Input: part model. Units: mm. Frame: model coordinates. A direction names the side the tool comes from. Give positions to 0.01 mm unless a question says otherwise; leave off trailing zeros. Order: outer loops, then holes, each group sorted by start corner. A loop starts at its lowest first (then second) coordinate and runs counter-clockwise, first axis right, second up. Notation, with made-up numbers: M 6.25,84.25 L 31.25,84.25 A27 ccw 31.25,108.25 Z; hole C 6,59 d8. An arc over 180 degrees is marked long. Use a Markdown table: item, result.
from build123d import *

# Parameters (mm, degrees)
SKETCH_1_W                 = 52.7
SKETCH_1_H                 = 13.9
EXTRUDE_1_DEPTH            = 11
SKETCH_2_W                 = 46.7
SKETCH_2_H                 = 10.9
CUT_EXTRUDE_1_DEPTH        = 9.5
SKETCH_3_W                 = 45.5
SKETCH_3_H                 = 1.5
EXTRUDE_2_DEPTH            = 8.4
SKETCH_4_W                 = 1
SKETCH_4_H                 = 7.5
CUT_EXTRUDE_2_DEPTH        = 51.794807806
CUT_EXTRUDE_3_DEPTH        = 3
PATTERN_LINEAR_1_COUNT     = 4
PATTERN_LINEAR_1_PITCH     = 5
CUT_EXTRUDE_4_DEPTH        = 3
PATTERN_LINEAR_2_COUNT     = 4
PATTERN_LINEAR_2_PITCH     = 5
SKETCH_7_W                 = 3.6
SKETCH_7_H                 = 5.5
CUT_EXTRUDE_5_DEPTH        = 32.757400712
SKETCH_8_W                 = 50.7
SKETCH_8_H                 = 11.9
CUT_EXTRUDE_6_DEPTH        = 0.5
SKETCH_9_R                 = 2.1
CUT_EXTRUDE_7_DEPTH        = 5
PATTERN_LINEAR_3_COUNT     = 5
PATTERN_LINEAR_3_PITCH     = 5.08
PATTERN_LINEAR_3_COL_COUNT = 5
PATTERN_LINEAR_3_COL_PITCH = 5.08
SKETCH_10_W                = 47.5
SKETCH_10_H                = 2
CUT_EXTRUDE_8_DEPTH        = 3
CUT_EXTRUDE_9_DEPTH        = 3


with BuildPart() as part:
    # Эскиз1 → Бобышка-Вытянуть1 (new body)
    with BuildSketch(Plane(origin=(0, 0, 0), x_dir=(1, 0, 0), z_dir=(0, 1, 0))):
        Rectangle(SKETCH_1_W, SKETCH_1_H)
    extrude(amount=EXTRUDE_1_DEPTH)

    # Эскиз2 → Вырез-Вытянуть1 (cut)
    with BuildSketch(Plane.XZ):
        Rectangle(SKETCH_2_W, SKETCH_2_H)
    extrude(amount=-CUT_EXTRUDE_1_DEPTH, mode=Mode.SUBTRACT)

    # Эскиз3 → Бобышка-Вытянуть2 (add)
    with BuildSketch(Plane.XZ):
        with Locations((0, 6.2)):
            Rectangle(SKETCH_3_W, SKETCH_3_H)
    extrude(amount=EXTRUDE_2_DEPTH)

    # Эскиз4 → Вырез-Вытянуть2 (cut, through all)
    with BuildSketch(Plane(origin=(22.75, 0, 0), x_dir=(0, 0, -1), z_dir=(1, 0, 0))):
        with Locations((-6.75, -5.15)):
            Rectangle(SKETCH_4_W, SKETCH_4_H)
    extrude(amount=-CUT_EXTRUDE_2_DEPTH, mode=Mode.SUBTRACT)

    # Эскиз5 → Вырез-Вытянуть3 (cut)
    with BuildSketch(Plane.XY.offset(6.25)):
        Polygon((-2.675, -1.4), (-2.675, -8), (-3.175, -8.5), (-3.675, -8.5), (-3.675, -9.5), (-1.375, -9.5), (-1.375, -8.5), (-1.875, -8.5), (-2.375, -8), (-2.375, -1.4), align=None)
    cut_extrude_3 = extrude(amount=-CUT_EXTRUDE_3_DEPTH, mode=Mode.SUBTRACT)

    # Линейный массив1: Вырез-Вытянуть3 ×4
    with Locations(*[(-i * PATTERN_LINEAR_1_PITCH, 0, 0) for i in range(1, PATTERN_LINEAR_1_COUNT)]):
        add(cut_extrude_3, mode=Mode.SUBTRACT)

    # Эскиз6 → Вырез-Вытянуть4 (cut)
    with BuildSketch(Plane.XY.offset(6.25)):
        Polygon((2.375, -1.4), (2.675, -1.4), (2.675, -8), (3.175, -8.5), (3.675, -8.5), (3.675, -9), (1.375, -9), (1.375, -8.5), (1.875, -8.5), (2.375, -8), align=None)
    cut_extrude_4 = extrude(amount=-CUT_EXTRUDE_4_DEPTH, mode=Mode.SUBTRACT)

    # Линейный массив2: Вырез-Вытянуть4 ×4
    with Locations(*[(i * PATTERN_LINEAR_2_PITCH, 0, 0) for i in range(1, PATTERN_LINEAR_2_COUNT)]):
        add(cut_extrude_4, mode=Mode.SUBTRACT)

    # Эскиз7 → Вырез-Вытянуть5 (cut, through all)
    with BuildSketch(Plane.XY.offset(6.95)):
        with Locations((-24.55, 1.75)):
            Rectangle(SKETCH_7_W, SKETCH_7_H)
        with Locations((24.55, 1.75)):
            Rectangle(SKETCH_7_W, SKETCH_7_H)
    extrude(amount=-CUT_EXTRUDE_5_DEPTH, mode=Mode.SUBTRACT)

    # Эскиз8 → Вырез-Вытянуть6 (cut)
    with BuildSketch(Plane(origin=(0, 11, 0), x_dir=(1, 0, 0), z_dir=(0, 1, 0))):
        Rectangle(SKETCH_8_W, SKETCH_8_H)
    extrude(amount=-CUT_EXTRUDE_6_DEPTH, mode=Mode.SUBTRACT)

    # Эскиз9 → Вырез-Вытянуть7 (cut)
    with BuildSketch(Plane(origin=(0, 10.5, 0), x_dir=(1, 0, 0), z_dir=(0, 1, 0))):
        with Locations(Location((0, 0, 0), (0, 0, 270))):
            Circle(SKETCH_9_R)
    cut_extrude_7 = extrude(amount=-CUT_EXTRUDE_7_DEPTH, mode=Mode.SUBTRACT)

    # Линейный массив3: Вырез-Вытянуть7 ×5
    with Locations(*[(-i * PATTERN_LINEAR_3_PITCH, 0, 0) for i in range(1, PATTERN_LINEAR_3_COUNT)]):
        add(cut_extrude_7, mode=Mode.SUBTRACT)

    # Линейный массив3 col: Вырез-Вытянуть7 ×5
    with Locations(*[(i * PATTERN_LINEAR_3_COL_PITCH, 0, 0) for i in range(1, PATTERN_LINEAR_3_COL_COUNT)]):
        add(cut_extrude_7, mode=Mode.SUBTRACT)

    # Эскиз10 → Вырез-Вытянуть8 (cut)
    with BuildSketch(Plane(origin=(0, 0, -6.95), x_dir=(-1, 0, 0), z_dir=(0, 0, -1))):
        Rectangle(SKETCH_10_W, SKETCH_10_H)
    extrude(amount=-CUT_EXTRUDE_8_DEPTH, mode=Mode.SUBTRACT)

    # Эскиз13 → Вырез-Вытянуть9 (cut)
    with BuildSketch(Plane.XY.offset(6.95)):
        Polygon((-26.35, 4.4), (-22.65, 4.4), (-22.35, -8.6), (-26.35, -8.6), align=None)
    cut_extrude_9 = extrude(amount=-CUT_EXTRUDE_9_DEPTH, mode=Mode.SUBTRACT)

    # Зеркальное отражение1: Вырез-Вытянуть9 across plane
    add(cut_extrude_9.mirror(Plane(origin=(0, 0, 0), x_dir=(0, 0, 1), z_dir=(1, 0, 0))), mode=Mode.SUBTRACT)


solid = part.part
1) Cut plane A-A on x = 16.5. Return loops of the section in (y, z).
Response values:
| item | result |
|---|---|
| outline | M -8.4,5.45 L 9.5,5.45 L 9.5,1.68 L 10.5,1.68 L 10.5,5.95 L 11,5.95 L 11,6.95 L -1.4,6.95 L -1.4,6.25 L -8.4,6.25 Z; M 1,-6.95 L 11,-6.95 L 11,-5.95 L 10.5,-5.95 L 10.5,-1.68 L 9.5,-1.68 L 9.5,-5.45 L 1,-5.45 Z |
2) Material intervals for line 1 (Z direction, x = -0.5, y = 7.25); line 2 (X direction, y = 7.5, z = -4.75); line 3 (Y direction, x = 8, z = -6), sorted ascending. Write a range as from..to.
Response values:
| item | result |
|---|---|
| line 1 | z = -6.95..-5.45, 5.45..6.95 |
| line 2 | x = -26.35..-23.35, 23.35..26.35 |
| line 3 | y = 1..11 |
3) Reachability of faces 1 (the face through (0, 0, 5.45)), 2 (the face through (0, 1, -6)), 3 (the face through (25, 4.5, 0)) from +Z, -Z, +X, -X, +Y, -Y: full face, straight path, thin tool, end or side. Return the list, or none.
Response values:
| item | result |
|---|---|
| face 1 | -Y |
| face 2 | -Z, +X, -X, -Y |
| face 3 | +Z, -Z, +X, -Y |
4) Mould query, pull axis X, two halves, no side actions, for faces 4 (the face through (26.35, 8, 0)), 5 (the face through (10, -5, 6.25)), 6 (the face through (18.457, 10.007, 0.969)). Classes: released by +X, released by -X, zero draft, split by the parting line, or undercut.
Response values:
| item | result |
|---|---|
| face 4 | released by +X |
| face 5 | zero draft |
| face 6 | undercut |
5) First-contact query: pin 1 Ø1.2 at (x, z) = (-10.5, -6) entering from -Y; pin 2 Ø6.5 at (x, z) = (0, 0) entering from -Y; pin 3 Ø5 at (x, y) = (-5, -4) entering from +Z; pin 4 Ø5 at (y, z) = (-3, -4.5) entering from -X. Flat tips, straight axial feed; report the tip coordinate or a pass-through.
Response values:
| item | result |
|---|---|
| pin 1 | stops at y = 1 |
| pin 2 | stops at y = 9.5 |
| pin 3 | stops at z = 6.25 |
| pin 4 | passes through |
6) Cut plane C-C on x = 5.08. Return loops of the section in (y, z).
Response values:
| item | result |
|---|---|
| outline | M -8.4,5.45 L 9.5,5.45 L 9.5,2.1 L 10.5,2.1 L 10.5,5.95 L 11,5.95 L 11,6.95 L -1.4,6.95 L -1.4,6.25 L -8.4,6.25 Z; M 1,-6.95 L 11,-6.95 L 11,-5.95 L 10.5,-5.95 L 10.5,-2.1 L 9.5,-2.1 L 9.5,-5.45 L 1,-5.45 Z |
7) Cut plane B-B on y = 5.5. Return loops of the section in (x, z).
Response values:
| item | result |
|---|---|
| outline | M -26.35,-6.95 L 26.35,-6.95 L 26.35,6.95 L -26.35,6.95 Z; hole M -23.35,-5.45 L 23.35,-5.45 L 23.35,5.45 L -23.35,5.45 Z |
